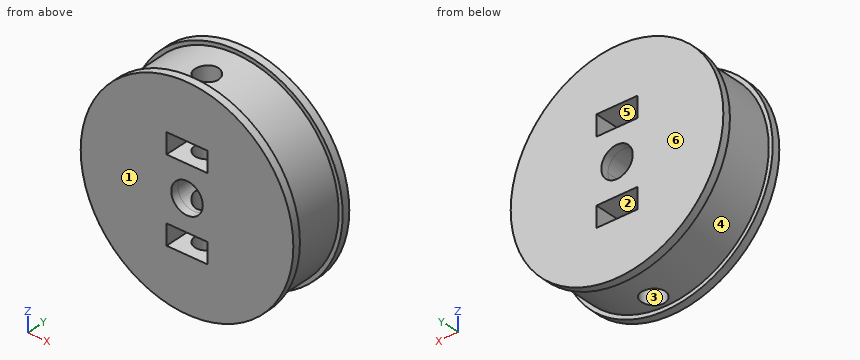
Autodesk Inventor part; units mm, degrees
ref_plane "YZ Plane" through (0, 0, 0) normal (1, 0, 0) x (0, 1, 0)
ref_plane "XZ Plane" through (0, 0, 0) normal (0, 1, 0) x (-1, 0, 0)
ref_plane "XY Plane" through (0, 0, 0) normal (0, 0, 1) x (1, 0, 0)
sketch "Эскиз1" plane through (0, 0, 0) normal (0, 1, 0) x (-1, 0, 0)
  circle A0 centre (0, 0) radius 13
  circle A1 centre (0, 0) radius 2
  dimension "d0" = 26
  dimension "d3" = 4
extrude "Выдавливание1" add sketch "Эскиз1" along normal blind 6.5
sketch "Эскиз2" plane through (0, 6.5, 0) normal (0, 1, 0) x (1, 0, 0)
  circle A0 centre (0, 0) radius 13.5
  dimension "d4" = 27
extrude "Выдавливание2" add sketch "Эскиз2" along normal blind 1
sketch "Эскиз3" plane through (0, 0, 0) normal (0, -1, 0) x (1, 0, 0)
  circle A0 centre (0, 0) radius 13.5
  dimension "d7" = 27
extrude "Выдавливание3" add sketch "Эскиз3" along normal blind 1
sketch "Эскиз4" plane through (0, 7.5, 0) normal (0, 1, 0) x (1, 0, 0)
  circle A0 centre (0, 0) radius 2
  line L0 (2.6, -6.6) -> (-2.6, -6.6)
  line L1 (-2.6, -6.6) -> (-2.6, -4)
  line L2 (-2.6, -4) -> (2.6, -4)
  line L3 (2.6, -4) -> (2.6, -6.6)
  line L4 (2.6, 4) -> (-2.6, 4)
  line L5 (-2.6, 4) -> (-2.6, 6.6)
  line L6 (-2.6, 6.6) -> (2.6, 6.6)
  line L7 (2.6, 6.6) -> (2.6, 4)
  dimension "d12" = 4
  dimension "d13" = 5.2
  dimension "d14" = 2.6
  dimension "d15" = 2.6
  dimension "d16" = 4
  dimension "d17" = 5.2
  dimension "d18" = 2.6
  dimension "d19" = 2.6
  dimension "d20" = 4
extrude "Выдавливание4" cut sketch "Эскиз4" against normal blind 8.75
ref_plane "РабПлоскость1" through (2.6, 7.5, -13) normal (0, 0, -1) x (-1, 0, 0)
sketch "Эскиз6" plane through (2.6, 7.5, -13) normal (0, 0, -1) x (-1, 0, 0)
  circle A0 centre (2.6, -5.5) radius 1.5
  line L0 (-10.9, -7.5) -> (16.1, -7.5)
  point P0 (2.6, -7.5)
  dimension "d24" = 3
  dimension "d25" = 2
extrude "Выдавливание5" cut sketch "Эскиз6" against normal blind 27
ref_plane "РабПлоскость2" through (13.4, 7.5, -4) normal (1, 0, 0) x (0, 0, -1)
properties part number "koleso"
Work out the finished part from the listing and answer in its coordinate system (mm). Face numbers are marked on the shaded views. A direction names the side the tool comes from. Coordinates: 2 decimals unless noted, no trailing zeros. Write each loop counter-clockwise with the first axis right and the second up, starting at its lowest first coordinate (ties: lowest second). Pieces come first, ordered by that corner, then holes.
1. The part is cut by section D-D, the plane x = 0. State how many separate pieces and enclosed holes the cut face has, and give its area (3 significant figures).
Results list:
separate pieces: 8
enclosed holes: 0
area: 94.4 mm2
2. For a pull along Y with two mould halves and no side action, classify the marked faces 1, 2, 3 and 4 as +Y half, -Y half, draft (parallel to the pull), parting line (faces both ways), or undercut.
Results list:
face 1: -Y half
face 2: draft
face 3: undercut
face 4: undercut
3. Consider line 1 along Z through (x, y) = (0, -0.3); line 2 along Y through (x, z) = (0, 3.35); line 3 along Z through (x, y) = (2.5, 3.25). Determine where each line is inside the solid, lowest interval first.
Results list:
line 1: z = -13.5 to -6.6, -4 to -2, 2 to 4, 6.6 to 13.5
line 2: y = -1 to 0.5, 3.5 to 7.5
line 3: z = -12.76 to -6.6, -4 to 4, 6.6 to 12.76
4. Flat-ended cylindrical pins translate along their axes: pin 1 (2.5 mm diameter, centred on x = -1, y = 4.5, fed in from -Z); pin 2 (5 mm diameter, centred on x = -5, y = 4, fed in from -Z); pin 3 (5 mm diameter, centred on x = 0, y = 2, fed in from +Z); pin 4 (3 mm diameter, centred on x = 9.5, y = 4, fed in from -Z). Find the tip coordinate at first contact, or state that the pin passes through.
Results list:
pin 1: stops at z = -13
pin 2: stops at z = -12.76
pin 3: stops at z = 13.5
pin 4: stops at z = -10.25
5. The part is cut by section A-A, the plane y = 5.75. Write down the section's boundary in (x, z).
Results list:
outline: circle Ø26 at (0, 0); hole (-2.6, -6.6) - (2.6, -6.6) - (2.6, -4) - (-2.6, -4) - close; hole (-2.6, 4) - (2.6, 4) - (2.6, 6.6) - (-2.6, 6.6) - close; hole circle Ø4 at (0, 0)
6. The part is cut by section B-B, the plane z = -3.5. Write down the section's boundary in (x, y), and give its area (3 significant figures).
Results list:
outline: (-13.04, -1) - (13.04, -1) - (13.04, 0) - (12.52, 0) - (12.52, 6.5) - (13.04, 6.5) - (13.04, 7.5) - (-13.04, 7.5) - (-13.04, 6.5) - (-12.52, 6.5) - (-12.52, 0) - (-13.04, 0) - close; hole circle Ø3 at (0, 2)
area: 208 mm2
7. The part is cut by section C-C, the plane y = 1. Write down the section's boundary in (x, z).
Results list:
outline: (-2.6, -6.6) - (-2.6, -4) - (-1.12, -4) - (-1.12, -1.66) arc R2 cw to (-1.12, 1.66) - (-1.12, 4) - (-2.6, 4) - (-2.6, 6.6) - (-1.12, 6.6) - (-1.12, 12.95) arc R13 ccw to (-1.12, -12.95) - (-1.12, -6.6) - close; (1.12, -12.95) arc R13 ccw to (1.12, 12.95) - (1.12, 6.6) - (2.6, 6.6) - (2.6, 4) - (1.12, 4) - (1.12, 1.66) arc R2 cw to (1.12, -1.66) - (1.12, -4) - (2.6, -4) - (2.6, -6.6) - (1.12, -6.6) - close
8. For the marked faces 5 and 6, determine the directions among +Z, -Z, +X, -X, +Y, -Y from which every point of the face is accessible in a straight line to the end or side of a thin tool.
Results list:
face 5: +Y, -Y
face 6: +Z, -Z, +X, -X, +Y
